```python
from build123d import *

# Parameters (mm, degrees)
ESBO_O1_W                                           = 20
ESBO_O1_H                                           = 70
FLANGE_BASE1_DEPTH                                  = 5
ARESTA_FLANGE1_STRIP_W                              = 30
ARESTA_FLANGE1_STRIP_H                              = 5
ARESTA_FLANGE1_STRIP_CUT_DEPTH                      = 70
ARESTA_FLANGE1_DEPTH                                = 70
ARESTA_FLANGE1_START                                = 5
ARESTA_FLANGE1_PROFILE_W                            = 90
ARESTA_FLANGE1_PROFILE_H                            = 162.6
ARESTA_FLANGE1_FLAT_DEPTH                           = 5
CORTE_EXTRUS_O1_DEPTH                               = 5
CORTE_EXTRUS_O2_DEPTH                               = 5
FILETE1_R                                           = 5
FILETE2_R                                           = 5
CORTE_EXTRUS_O3_REACH                               = 177.328
ESBO_O14_R                                          = 6.5
FILETE3_R                                           = 18
FILETE4_R                                           = 18
ESBO_O27_R                                          = 3.3
CORTE_EXTRUS_O4_DEPTH                               = 5
ESBO_O28_R                                          = 2.75
CORTE_EXTRUS_O5_DEPTH                               = 5
ESCAREADO_PARA_PARAFUSO_ALLEN_SEXTAVADO_D           = 3.4
ESCAREADO_PARA_PARAFUSO_ALLEN_SEXTAVADO_CSINK_D     = 7.72
ESCAREADO_PARA_PARAFUSO_ALLEN_SEXTAVADO_CSINK_ANGLE = 90
ESBO_O34_R                                          = 1.25
CORTE_EXTRUS_O6_DEPTH                               = 5


# Sheet-metal steps are written as plain solids
with BuildPart() as part:
    # Esboço1 → Flange-base1 (new body)
    with BuildSketch(Plane(origin=(0, 0, 0), x_dir=(1, 0, 0), z_dir=(0, 1, 0))):
        Rectangle(ESBO_O1_W, ESBO_O1_H)
    extrude(amount=-FLANGE_BASE1_DEPTH)

    # Aresta-Flange1 strip (across the edge) → Aresta-Flange1 strip cut (cut)
    with BuildSketch(Plane(origin=(-10, 0, -35), x_dir=(1, 0, 0), z_dir=(0, 0, 1))):
        with Locations((-10, -2.5)):
            Rectangle(ARESTA_FLANGE1_STRIP_W, ARESTA_FLANGE1_STRIP_H)
    extrude(amount=ARESTA_FLANGE1_STRIP_CUT_DEPTH, mode=Mode.SUBTRACT)

    # Aresta-Flange1 bend section (across the edge) → Aresta-Flange1 (add)
    with BuildSketch(Plane(origin=(-10, 0, -35), x_dir=(1, 0, 0), z_dir=(0, 0, 1))):
        with BuildLine():
            Line((-5, 5), (0, 5))
            ThreePointArc((0, 5), (1.464466094, 1.464466094), (5, 0))
            Line((5, 0), (5, -5))
            ThreePointArc((5, -5), (-2.071067812, -2.071067812), (-5, 5))
        make_face()
    extrude(amount=ARESTA_FLANGE1_DEPTH)

    # Aresta-Flange1 profile (on flange) → Aresta-Flange1 flat (add)
    with BuildSketch(Plane.ZY.offset(10).offset(ARESTA_FLANGE1_START)):
        with Locations((0, 86.3)):
            Rectangle(ARESTA_FLANGE1_PROFILE_W, ARESTA_FLANGE1_PROFILE_H)
    extrude(amount=-ARESTA_FLANGE1_FLAT_DEPTH)

    # Esboço11 → Corte-extrusão1 (cut)
    with BuildSketch(Plane(origin=(-10, 0, 0), x_dir=(0, 0, -1), z_dir=(1, 0, 0))):
        with BuildLine():
            Line((35, 5.5), (35, 16.756560302))
            ThreePointArc((35, 16.756560302), (35.785363848, 19.446698236), (37.894736842, 21.291741339))
            ThreePointArc((37.894736842, 21.291741339), (40.139210452, 22.371640143), (42.352941176, 23.513235294))
            ThreePointArc((42.352941176, 23.513235294), (44.287464629, 25.352521223), (45, 27.925))
            Line((45, 27.925), (45, 5))
            Line((45, 5), (35, 5))
            Line((35, 5), (35, 5.5))
        make_face()
    extrude(amount=-CORTE_EXTRUS_O1_DEPTH, mode=Mode.SUBTRACT)

    # Esboço12 → Corte-extrusão2 (cut)
    with BuildSketch(Plane(origin=(-10, 0, 0), x_dir=(0, 0, -1), z_dir=(1, 0, 0))):
        with BuildLine():
            Line((-45, 5), (-35, 5))
            Line((-35, 5), (-35, 20.009380241))
            ThreePointArc((-35, 20.009380241), (-40.077219356, 22.340780151), (-45, 24.982713659))
            Line((-45, 24.982713659), (-45, 5))
        make_face()
    extrude(amount=-CORTE_EXTRUS_O2_DEPTH, mode=Mode.SUBTRACT)

    # Filete1
    filete1_edges = [part.edges().sort_by_distance(p)[0] for p in [
        (-12.5, 20.009380241, 35),
    ]]
    fillet(filete1_edges, radius=FILETE1_R)

    # Filete2
    filete2_edges = [part.edges().sort_by_distance(p)[0] for p in [
        (-12.5, 24.982713659, 45),
    ]]
    fillet(filete2_edges, radius=FILETE2_R)

    # Esboço14 → Corte-extrusão3 (cut, up to next)
    with BuildSketch(Plane.ZY.offset(15), mode=Mode.PRIVATE) as corte_extrus_o3_sk1:
        with Locations(Location((-33, 102.925, 0), (0, 0, 270))):
            Circle(ESBO_O14_R)
    corte_extrus_o3_tool1 = extrude(corte_extrus_o3_sk1.sketch, amount=-CORTE_EXTRUS_O3_REACH, mode=Mode.PRIVATE) & part.part
    # Esboço14 → Corte-extrusão3 (cut, up to next)
    with BuildSketch(Plane.ZY.offset(15), mode=Mode.PRIVATE) as corte_extrus_o3_sk2:
        with Locations(Location((33, 102.925, 0), (0, 0, 270))):
            Circle(ESBO_O14_R)
    corte_extrus_o3_tool2 = extrude(corte_extrus_o3_sk2.sketch, amount=-CORTE_EXTRUS_O3_REACH, mode=Mode.PRIVATE) & part.part
    add(corte_extrus_o3_tool1.solids().sort_by_distance((-15, 102.925, -33))[0], mode=Mode.SUBTRACT)
    add(corte_extrus_o3_tool2.solids().sort_by_distance((-15, 102.925, 33))[0], mode=Mode.SUBTRACT)

    # Filete3
    filete3_edges = [part.edges().sort_by_distance(p)[0] for p in [
        (-12.5, 167.6, 45),
    ]]
    fillet(filete3_edges, radius=FILETE3_R)

    # Filete4
    filete4_edges = [part.edges().sort_by_distance(p)[0] for p in [
        (-12.5, 167.6, -45),
    ]]
    fillet(filete4_edges, radius=FILETE4_R)

    # Esboço27 → Corte-extrusão4 (cut)
    with BuildSketch(Plane.ZY.offset(15)):
        with Locations(Location((7.5, 155.925, 0), (0, 0, 270))):
            Circle(ESBO_O27_R)
        with Locations(Location((-7.5, 155.925, 0), (0, 0, 270))):
            Circle(ESBO_O27_R)
    extrude(amount=-CORTE_EXTRUS_O4_DEPTH, mode=Mode.SUBTRACT)

    # Esboço28 → Corte-extrusão5 (cut)
    with BuildSketch(Plane(origin=(0, 0, 0), x_dir=(1, 0, 0), z_dir=(0, 1, 0))):
        with Locations(Location((0, 13, 0), (0, 0, 270))):
            Circle(ESBO_O28_R)
        with Locations(Location((0, -13, 0), (0, 0, 270))):
            Circle(ESBO_O28_R)
    extrude(amount=-CORTE_EXTRUS_O5_DEPTH, mode=Mode.SUBTRACT)

    # Escareado para parafuso Allen sextavado escareado de M32 (through all)
    with Locations(Plane(origin=(-10, 0, 0), x_dir=(0, 0, -1), z_dir=(1, 0, 0))):
        with Locations((-15.5, 87.425), (-15.5, 118.425), (15.5, 118.425), (15.5, 87.425)):
            CounterSinkHole(ESCAREADO_PARA_PARAFUSO_ALLEN_SEXTAVADO_D / 2, ESCAREADO_PARA_PARAFUSO_ALLEN_SEXTAVADO_CSINK_D / 2, counter_sink_angle=ESCAREADO_PARA_PARAFUSO_ALLEN_SEXTAVADO_CSINK_ANGLE)

    # Esboço34 → Corte-extrusão6 (cut)
    with BuildSketch(Plane(origin=(-10, 0, 0), x_dir=(0, 0, -1), z_dir=(1, 0, 0))):
        with Locations(Location((-33, 112.924999999, 0), (0, 0, 90))):
            Circle(ESBO_O34_R)
        with Locations(Location((-33, 92.924999999, 0), (0, 0, 90))):
            Circle(ESBO_O34_R)
        with Locations(Location((33, 112.924999999, 0), (0, 0, 90))):
            Circle(ESBO_O34_R)
        with Locations(Location((33, 92.924999999, 0), (0, 0, 90))):
            Circle(ESBO_O34_R)
    extrude(amount=-CORTE_EXTRUS_O6_DEPTH, mode=Mode.SUBTRACT)


solid = part.part
```
CAD build for the part. Positions are in the model's coordinates, mm. A direction names the side the tool comes from. Coordinates: 2 decimals unless noted, no trailing zeros. Order: outer loops, then holes, each group sorted by start corner. A loop starts at its lowest first (then second) coordinate and runs counter-clockwise, first axis right, second up. Notation, with made-up numbers: M 28.25,66 L 49.25,66 A13 cw 49.25,91 Z; hole C 37.5,46 d3. An arc over 180 degrees is marked long. Write each question's results on one line, items separated by ' | '. Start each with the question number.
Q1. Cut at B-B (y = 100.5). List the corners of the cut face in (x, z), then the cut area to 3 significant figures.
Q2. Cut at D-D (y = 65.5). List the corners of the cut face in (x, z).
Q3. Which spindle directions (+Z, -Z, +X, -X, +Y, -Y) get a long thin tool onto all of the face, cutting with end or side? Do faces 4 (the flat face through (-5, -2, -35)), 5 (the flat face through (10, -2, 0)). Say none if no direction does.
Q4. Cut at A-A (x = 0). List the corners of the cut face in (y, z).
Q5. Pull direction Z, two halves, no side cores. Call faces 1 (the flat face through (2, 0, 0)), 2 (the cylindrical face through (-12.535, 103.771, -26.555)), 3 (the cylindrical face through (-12.54, 25.32, 44.27)): +Z half, -Z half, draft (parallel to the pull), parting line (faces both ways), or undercut.
Q6. Flat gauge pins, fed straight in: P1, Ø6.5, axis at x = 0, z = 13, coming from the +Y side; P2, Ø2, axis at y = 112.925, z = -33, coming from the +X side; P3, Ø3, axis at y = 101, z = 1, coming from the +X side. Where does each tip first touch, or does it go through?
Q7. Cut at C-C (z = 7.5). List the corners of the cut face in (x, y) (3 decimals), then the cut area to 3 significant figures.
Q8. Drill centre lines: probe 1 along Y at (x, z) = (-13.7, 15.5) (3 decimals); probe 2 along Y at (x, z) = (-13.4, 15.5) (3 decimals); probe 3 along X at (y, z) = (30, -3). Where is each one in solid material? Low to high. Write a range as from..to.
Found:
1) outline: M -15,-45 L -10,-45 L -10,-39.03 L -15,-39.03 Z; M -15,-26.97 L -10,-26.97 L -10,26.97 L -15,26.97 Z; M -15,39.03 L -10,39.03 L -10,45 L -15,45 Z | area: 329 mm²
2) outline: M -15,-45 L -10,-45 L -10,45 L -15,45 Z
3) face 4: -Z, +X, -X, -Y | face 5: +Z, -Z, +X, +Y, -Y
4) outline: M -5,-35 L 0,-35 L 0,-15.75 L -5,-15.75 Z; M -5,-10.25 L 0,-10.25 L 0,10.25 L -5,10.25 Z; M -5,15.75 L 0,15.75 L 0,35 L -5,35 Z
5) face 1: draft | face 2: undercut | face 3: +Z half
6) P1: y = 0 | P2: through | P3: x = -10
7) outline: M -15,5 A10 ccw -5,-5 L 10,-5 L 10,0 L -5,0 A5 cw -10,5 L -10,152.625 L -15,152.625 Z; M -15,159.225 L -10,159.225 L -10,167.6 L -15,167.6 Z | area: 914 mm²
8) probe 1: 0.069..85.725, 89.125..116.725, 120.125..167.6 | probe 2: -0.426..85.725, 89.125..116.725, 120.125..167.6 | probe 3: -15..-10
